The drawing under review shows one solid part. Ordinate dimensions are in mm from its lowest x, y, z. Coordinates: 2 decimals unless noted, no trailing zeros. Loops run counter-clockwise (first coordinate to the right, second up) from the corner with the lowest first, then second, coordinate; pieces in that order, holes last. Notation, with made-up numbers: M 50,-9.5 L 68,-9.5 A26 ccw 68,20.5 Z; hole C 27,53 d1. An arc over 180 degrees is marked long. Use one line per item in the form item = value.
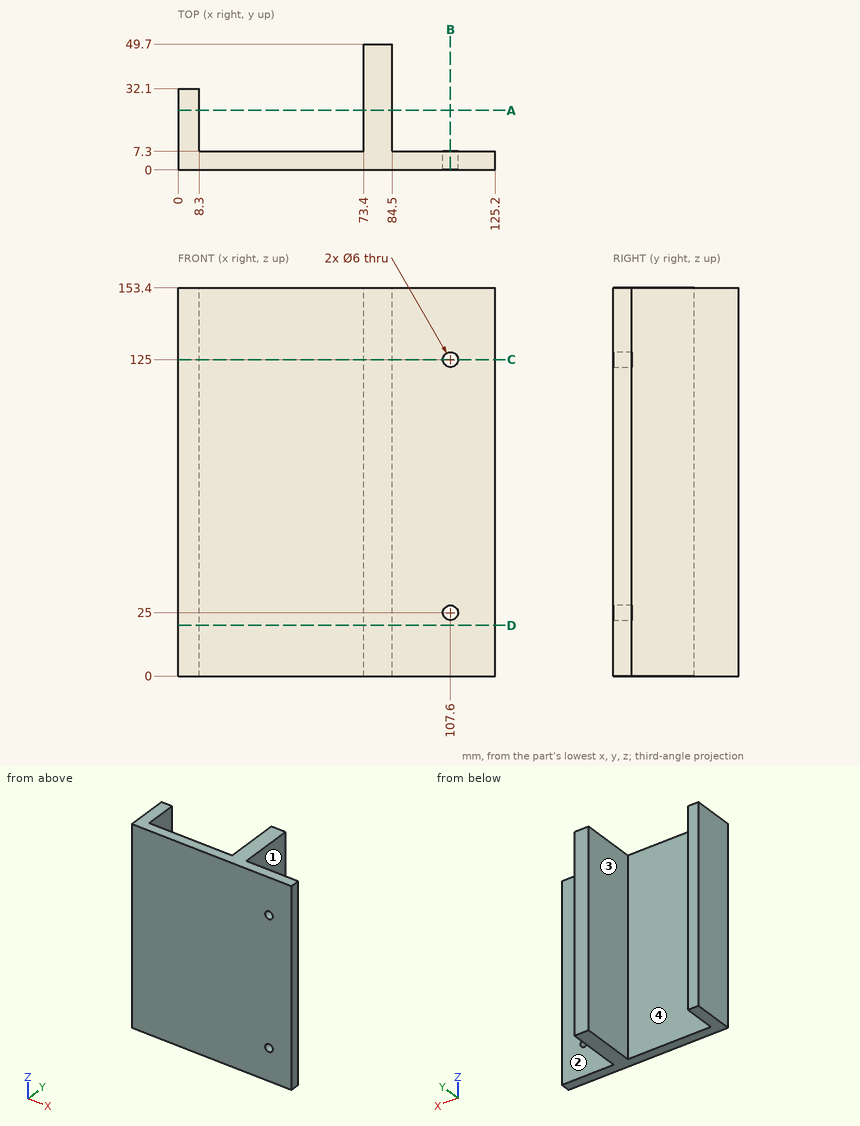
1. Consider section B-B on x = 107.6. Write out the cut boundary in (y, z).
Computed values:
outline = M 0,0 L 7.3,0 L 7.3,22 L 0,22 Z; M 0,28 L 7.3,28 L 7.3,122 L 0,122 Z; M 0,128 L 7.3,128 L 7.3,153.4 L 0,153.4 Z
2. Wall thickness on line 1 along X through (y, z) = (17, 78); line 2 along X through (y, z) = (4.5, 25); line 3 along Z through (x, y) = (107, 4): over which ranges is each line inside the solid? List them lowest first. Write a range as from..to.
Computed values:
line_1 = 0..8.3, 73.4..84.5
line_2 = 0..104.6, 110.6..125.2
line_3 = 0..22.06, 27.94..122.06, 127.94..153.4
3. Consider section C-C on z = 125. Write out the cut boundary in (x, y), plus the area to 3 significant figures.
Computed values:
outline = M 0,0 L 104.6,0 L 104.6,7.3 L 84.5,7.3 L 84.5,49.7 L 73.4,49.7 L 73.4,7.3 L 8.3,7.3 L 8.3,32.1 L 0,32.1 Z; M 110.6,0 L 125.2,0 L 125.2,7.3 L 110.6,7.3 Z
area = 1,550 mm2
4. Draft analysis for pull direction X (two halves, no side actions). For the marked faces 1, 2, 3 and 4, state which applies: +X half, -X half, draft (parallel to the pull), parting line (faces both ways), or undercut.
Computed values:
face_1 = +X half
face_2 = draft
face_3 = undercut
face_4 = undercut
5. Consider section D-D on z = 20. Write out the cut boundary in (x, y), plus the area to 3 significant figures.
Computed values:
outline = M 0,0 L 125.2,0 L 125.2,7.3 L 84.5,7.3 L 84.5,49.7 L 73.4,49.7 L 73.4,7.3 L 8.3,7.3 L 8.3,32.1 L 0,32.1 Z
area = 1,590 mm2
6. Consider section A-A on y = 23.5. Write out the cut boundary in (x, z).
Computed values:
outline = M 0,0 L 8.3,0 L 8.3,153.4 L 0,153.4 Z; M 73.4,0 L 84.5,0 L 84.5,153.4 L 73.4,153.4 Z
7. For pin 1 Ø12.5 at (y, z) = (24, 42.5) entering from +X; pin 2 Ø2.5 at (x, z) = (5.5, 115) entering from +Y, all flat-tipped, find the tip position at first contact; note any pin that passes through.
Computed values:
pin_1 = 84.5
pin_2 = 32.1
